Geometry check sheet. Reference: the model listing, model coordinates, mm. Face numbers are marked on the shaded views. Coordinates: 2 decimals unless noted, no trailing zeros. Write each loop counter-clockwise with the first axis right and the second up, starting at its lowest first coordinate (ties: lowest second). Pieces come first, ordered by that corner, then holes. Notation, with made-up numbers: (79, 35.25) -> (126, 35.25) arc R25 cw to (126, 70.25) -> close; hole circle Ø9 at (58, 21). An arc over 180 degrees is marked (long way). Answer in a Markdown table with one row per item. Add a question column.
1. Mould release check, pull along Y, two halves, no side actions. Record for the marked faces 1 and 2: pulls with the +Y half, pulls with the -Y half, needs draft (parallel to the pull), parting line crosses it, or undercut.
2. Scan lines: L1, parallel to Y at x = 6.25, z = 2.35; L2, parallel to Z at x = 7.5, y = -26.5; L3, parallel to X at y = -29.5, z = 2.75. Record each from-to range of solid material in increasing order. Write a range as from..to.
3. Depth check by flat-ended pin: P1, Ø0.7, axis at x = 26, z = 1, coming from the +Y side (3 decimals); P2, Ø1.6, axis at x = 12.5, z = 3, coming from the -Y side; P3, Ø0.6, axis at y = -29.5, z = 2.5, coming from the +X side; P4, Ø2, axis at y = -12, z = 3, coming from the -X side. Enter the tip coordinate at first touch or a pass-through.
4. Cross-section at A-A on x = 9. Record the cut outline in (y, z) (3 decimals), and give its area (3 significant figures).
5. Cross-section at C-C on y = -12. Record the cut outline in (x, z) (3 decimals).
6. Cross-section at B-B on y = -23. Record the cut outline in (x, z) (3 decimals), and give its area (3 significant figures).
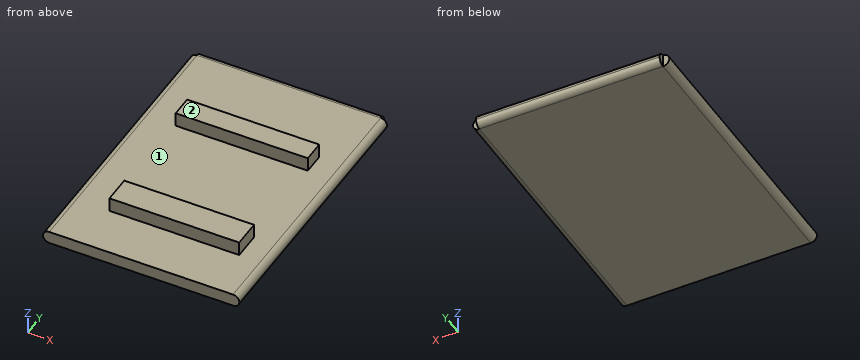
```python
from build123d import *

# Parameters (mm, degrees)
F0_W     = 25.7
F0_H     = 38.7
F1_DEPTH = 1.77
F4_DEPTH = 38.7
F5_DEPTH = 25.7
F6_W     = 18.1557917967
F6_H     = 3.8920287043
F6_W_2   = 18.4808271006
F6_H_2   = 2.9954407364
F7_DEPTH = 2


with BuildPart() as f1:
    # F0 (on Top) → F1 (new body)
    with BuildSketch(Plane.XY):
        with Locations((12.85, -19.35)):
            Rectangle(F0_W, F0_H)
    extrude(amount=F1_DEPTH)

    # F2 (on face) → F4 (join)
    with BuildSketch(Plane.XZ.offset(38.7)):
        with BuildLine():
            ThreePointArc((25.7, 0), (26.3257895014, 0.2592104986), (26.585, 0.885))
            ThreePointArc((26.585, 0.885), (26.3257895014, 1.5107895014), (25.7, 1.77))
            Line((25.7, 1.77), (25.7, 0))
        make_face()
        with BuildLine():
            Line((25.7, 0), (25.7, 1.77))
            ThreePointArc((25.7, 1.77), (24.815, 0.885), (25.7, 0))
        make_face()
        with BuildLine():
            Line((0, 0), (0, 1.77))
            ThreePointArc((0, 1.77), (-0.885, 0.885), (0, 0))
        make_face()
    extrude(amount=-F4_DEPTH)

    # F3 (on face) → F5 (join)
    with BuildSketch(Plane.YZ.offset(25.7)):
        with BuildLine():
            ThreePointArc((0, 0), (0.6257895014, 0.2592104986), (0.885, 0.885))
            ThreePointArc((0.885, 0.885), (0.6257895014, 1.5107895014), (0, 1.77))
            Line((0, 1.77), (0, 0))
        make_face()
        with BuildLine():
            Line((0, 0), (0, 1.77))
            ThreePointArc((0, 1.77), (-0.885, 0.885), (0, 0))
        make_face()
    extrude(amount=-F5_DEPTH)

    # F6 (on face) → F7 (join)
    with BuildSketch(Plane.XY.offset(1.77)):
        with Locations((13.7009262107, -29.6595497057)):
            Rectangle(F6_W, F6_H)
        with Locations((13.3267915808, -11.7375161499)):
            Rectangle(F6_W_2, F6_H_2)
    extrude(amount=F7_DEPTH)


solid = f1.part
```
Results found:
| question | item | result |
|---|---|---|
| 1 | face 1 | undercut |
| 1 | face 2 | needs draft |
| 2 | L1 | y = -31.61..-27.71, -13.24..-10.24 |
| 2 | L2 | z = 0..1.77 |
| 2 | L3 | x = 4.62..22.78 |
| 3 | P1 | stops at y = 0.885 |
| 3 | P2 | stops at y = -31.61 |
| 3 | P3 | stops at x = 22.78 |
| 3 | P4 | stops at x = 4.09 |
| 4 | outline | (-38.7, 0) -> (0, 0) arc R0.885 ccw to (0, 1.77) -> (-10.24, 1.77) -> (-10.24, 3.77) -> (-13.235, 3.77) -> (-13.235, 1.77) -> (-27.714, 1.77) -> (-27.714, 3.77) -> (-31.606, 3.77) -> (-31.606, 1.77) -> (-38.7, 1.77) -> close |
| 4 | area | 83.5 mm^2 |
| 5 | outline | (0, 0) -> (25.7, 0) arc R0.885 ccw to (25.7, 1.77) -> (22.567, 1.77) -> (22.567, 3.77) -> (4.086, 3.77) -> (4.086, 1.77) -> (0, 1.77) arc R0.885 ccw to start |
| 6 | outline | (0, 0) -> (25.7, 0) arc R0.885 ccw to (25.7, 1.77) -> (0, 1.77) arc R0.885 ccw to start |
| 6 | area | 47.9 mm^2 |
